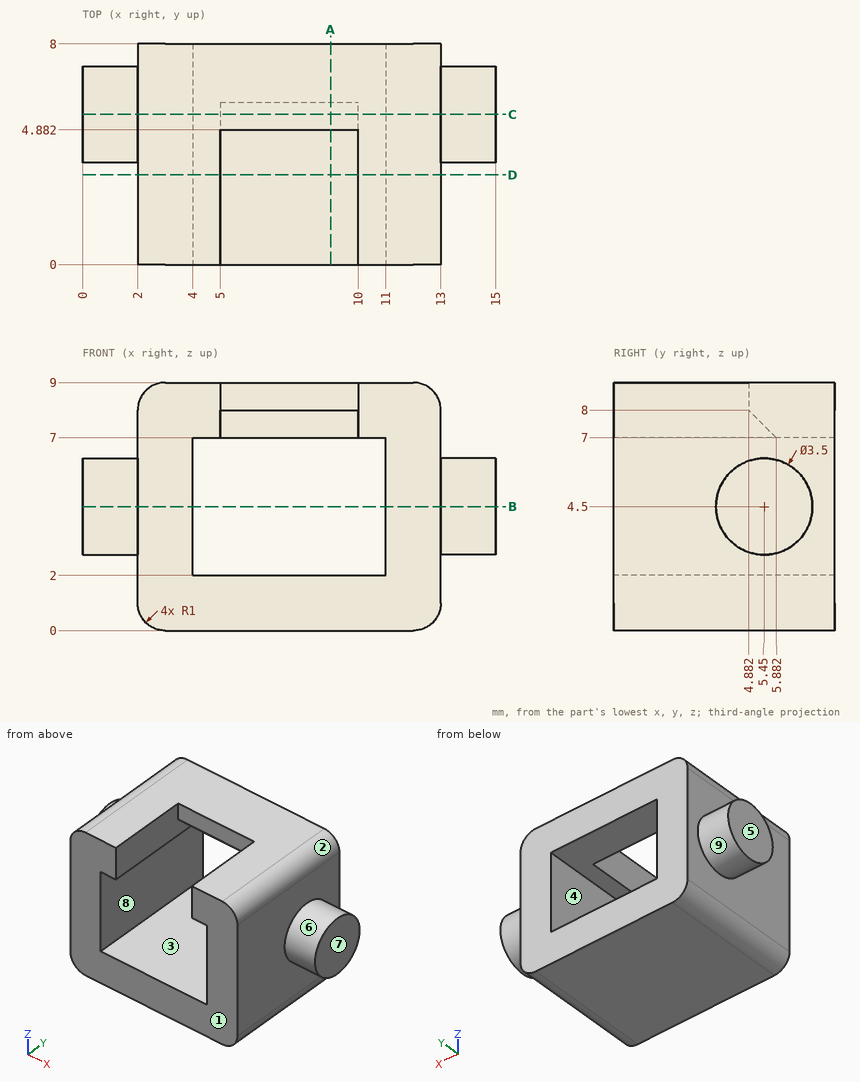
Could you check a few things on this drawing? It's one solid part, dimensions in mm from its lowest x, y, z. A direction names the side the tool comes from. Round coordinates to 2 decimals unless told otherwise and drop trailing zeros. Order: outer loops, then holes, each group sorted by start corner. A loop starts at its lowest first (then second) coordinate and runs counter-clockwise, first axis right, second up. Notation, with made-up numbers: M 1.25,-23 L 41.25,-23 A19 ccw 41.25,13 Z; hole C 16,-4 d11. An arc over 180 degrees is marked long. Use a Markdown table: item, result.
1) Imagine slicing it at B-B (z = 4.5). List the corners of the cut face in (x, y) for me, then the cut area to 3 significant figures.
Geometry says:
| item | result |
|---|---|
| outline | M 0,3.7 L 2,3.7 L 2,0 L 4,0 L 4,8 L 2,8 L 2,7.2 L 0,7.2 Z; M 11,0 L 13,0 L 13,3.7 L 15,3.7 L 15,7.2 L 13,7.2 L 13,8 L 11,8 Z |
| area | 46.0 mm² |
2) On a 3-axis mill with a long thin cutter (end or side, diameter ignored), from which of +Z, -Z, +X, -X, +Y, -Y can I reach the whole of each face in a straight line? I mean the marked faces 5, 6, 7, 8 and 9. Say none if no direction works.
Geometry says:
| item | result |
|---|---|
| face 5 | +Z, -Z, -X, +Y, -Y |
| face 6 | +X |
| face 7 | +Z, -Z, +X, +Y, -Y |
| face 8 | +Y, -Y |
| face 9 | -X |
3) I'm going to push flat-ended pins straight in: P1, Ø1, axis at y = 4, z = 1.5, coming from the -X side; P2, Ø2, axis at y = 2.5, z = 6, coming from the +X side; P3, Ø3, axis at x = 9, y = 1, coming from the +Z side; P4, Ø1.1, axis at x = 8.5, z = 8.5, coming from the -Y side. Where does each tip first touch, or does it pass through?
Geometry says:
| item | result |
|---|---|
| P1 | stops at x = 2 |
| P2 | stops at x = 13 |
| P3 | stops at z = 9 |
| P4 | stops at y = 4.88 |
4) Imagine slicing it at C-C (y = 5.45). List the corners of the cut face in (x, z) for me.
Geometry says:
| item | result |
|---|---|
| outline | M 0,2.75 L 2,2.75 L 2,1 A1 ccw 3,0 L 12,0 A1 ccw 13,1 L 13,2.75 L 15,2.75 L 15,6.25 L 13,6.25 L 13,8 A1 ccw 12,9 L 3,9 A1 ccw 2,8 L 2,6.25 L 0,6.25 Z; hole M 4,2 L 11,2 L 11,7 L 10,7 L 10,7.43 L 5,7.43 L 5,7 L 4,7 Z |
5) Imagine slicing it at D-D (y = 3.25). List the corners of the cut face in (x, z) for me.
Geometry says:
| item | result |
|---|---|
| outline | M 2,1 A1 ccw 3,0 L 12,0 A1 ccw 13,1 L 13,8 A1 ccw 12,9 L 10,9 L 10,7 L 11,7 L 11,2 L 4,2 L 4,7 L 5,7 L 5,9 L 3,9 A1 ccw 2,8 Z |
6) Imagine slicing it at A-A (x = 9). List the corners of the cut face in (y, z) for me.
Geometry says:
| item | result |
|---|---|
| outline | M 0,0 L 8,0 L 8,2 L 0,2 Z; M 4.88,8 L 5.88,7 L 8,7 L 8,9 L 4.88,9 Z |
7) If I drill on line 1 along X through (y, z) = (5.75, 6.75); line 2 along Z through (x, y) = (4.5, 4.25); line 3 along X through (y, z) = (5, 4), over which ranges is the centre line in solid material (lowest first)?
Geometry says:
| item | result |
|---|---|
| line 1 | x = 2 to 4, 11 to 13 |
| line 2 | z = 0 to 2, 7 to 9 |
| line 3 | x = 0 to 4, 11 to 15 |
8) If we mould it in two halves opening along Z, with no side actions, what happens to the marked faces 1, 2, 3 and 4? For each: +Z half, -Z half, draft (parallel to the pull), parting line (faces both ways), or undercut.
Geometry says:
| item | result |
|---|---|
| face 1 | draft |
| face 2 | +Z half |
| face 3 | undercut |
| face 4 | undercut |
